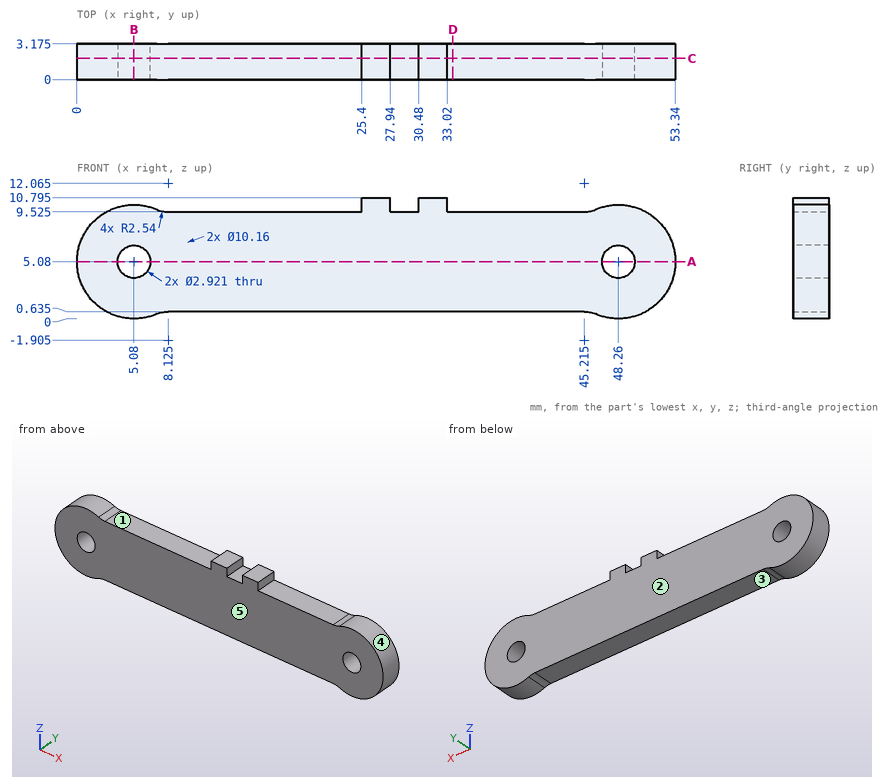
The figure shows three views and two pictorial views of one solid part (mm, origin at its lowest corner). Answer the questions. A direction names the side the tool comes from. Round coordinates to 2 decimals unless told otherwise and drop trailing zeros. Write each loop counter-clockwise with the first axis right and the second up, starting at its lowest first coordinate (ties: lowest second). Pieces come first, ordered by that corner, then holes. Notation, with made-up numbers: M 18,-10 L 28,-10 A22 cw 28,-1 Z; hole C 50,23.25 d2. An arc over 180 degrees is marked long. Write each question's results on one line, items separated by ' | '. Start each with the question number.
(1) Determine the mould class of the marked faces 4 and 5 for opening direction X: +X half, -X half, draft (parallel to the pull), parting line (faces both ways), or undercut.
(2) The part is cut by section A-A, the plane z = 5.08. Write down the section's boundary in (x, y) (1 decimal), and give its area (3 significant figures).
(3) The part is cut by section B-B, the plane x = 5.08. Write down the section's boundary in (y, z) (1 decimal).
(4) Each of these flat-tipped pins is pushed along its axis until it touches: P1, Ø0.6, axis at y = 1.5, z = 10, coming from the +X side (1 decimal); P2, Ø1, axis at x = 32, y = 2, coming from the -Z side (3 decimals); P3, Ø1.6, axis at x = 16.5, y = 1, coming from the +Z side (3 decimals). Where does it stop, or does it pass through?
(5) Find the intervals of material crossed by line 1 (X direction, y = 1.65, z = 5.08); line 2 (Z direction, x = 48.26, y = 1.25); line 3 (X direction, y = 2, z = 4) (1 decimal), in increasing order.
(6) The part is cut by section C-C, the plane y = 1.9. Write down the section's boundary in (x, z) (1 decimal).
(7) The part is cut by section D-D, the plane x = 33.5. Write down the section's boundary in (y, z) (1 decimal), and give its area (3 significant figures).
(8) For the marked faces 1, 2 and 3, determine the directions among +Z, -Z, +X, -X, +Y, -Y from which every point of the face is accessible in a straight line to the end or side of a thin tool.
Worked answers:
1) face 4: undercut | face 5: draft
2) outline: M 0,0 L 3.6,0 L 3.6,3.2 L 0,3.2 Z; M 6.5,0 L 46.8,0 L 46.8,3.2 L 6.5,3.2 Z; M 49.7,0 L 53.3,0 L 53.3,3.2 L 49.7,3.2 Z | area: 151 mm²
3) outline: M 0,0 L 3.2,0 L 3.2,3.6 L 0,3.6 Z; M 0,6.5 L 3.2,6.5 L 3.2,10.2 L 0,10.2 Z
4) P1: stops at x = 50.4 | P2: stops at z = 0.635 | P3: stops at z = 9.525
5) line 1: x = 0 to 3.62, 6.54 to 46.8, 49.72 to 53.34 | line 2: z = 0 to 3.62, 6.54 to 10.16 | line 3: x = 0.1 to 4.1, 6.1 to 47.3, 49.2 to 53.2
6) outline: M 7.1,0.4 A2.5 cw 8.1,0.6 L 45.2,0.6 A2.5 cw 46.2,0.4 A5.1 ccw long 46.2,9.7 A2.5 cw 45.2,9.5 L 33,9.5 L 33,10.8 L 30.5,10.8 L 30.5,9.5 L 27.9,9.5 L 27.9,10.8 L 25.4,10.8 L 25.4,9.5 L 8.1,9.5 A2.5 cw 7.1,9.7 A5.1 ccw long Z; hole C 5.1,5.1 d2.9; hole C 48.3,5.1 d2.9
7) outline: M 0,0.6 L 3.2,0.6 L 3.2,9.5 L 0,9.5 Z | area: 28.2 mm²
8) face 1: +Z, +Y, -Y | face 2: +Z, -Z, +X, -X, +Y | face 3: -Z, +Y, -Y
